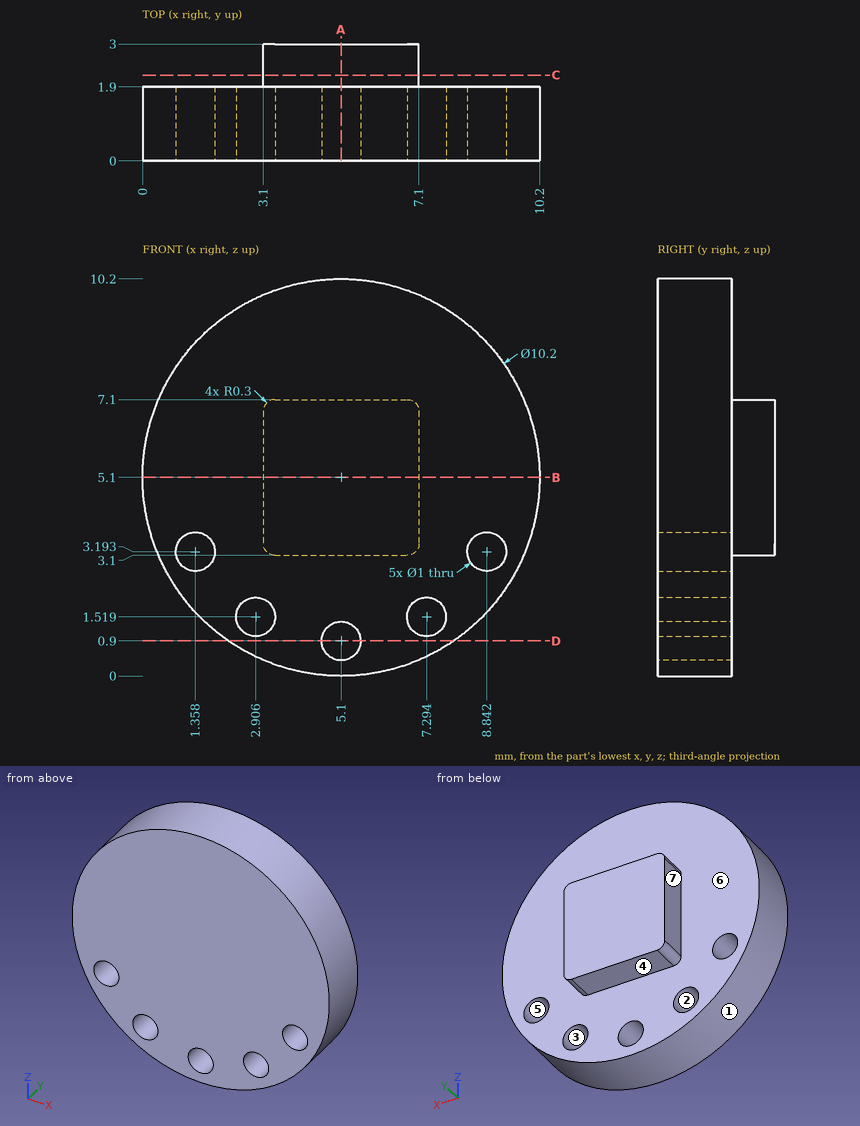
The figure shows three views and two pictorial views of one solid part (mm, origin at its lowest corner). Answer the questions. A direction names the side the tool comes from. Round coordinates to 2 decimals unless told otherwise and drop trailing zeros. Write each loop counter-clockwise with the first axis right and the second up, starting at its lowest first coordinate (ties: lowest second). Pieces come first, ordered by that corner, then holes. Notation, with made-up numbers: M 87,-2 L 136,-2 A13 cw 136,19 Z; hole C 83.25,8.25 d1. An arc over 180 degrees is marked long. Use a Markdown table: item, result.
1) A flat-ended cylindrical pin translates along its axis: pin 1 (1.5 mm diameter, centred on x = 4, y = 2.5, fed in from +Z). Find the tip coordinate at first contact, or state that the pin passes through.
Taken from the geometry:
| item | result |
|---|---|
| pin 1 | stops at z = 10.16 |
2) Consider line 1 (X direction, y = 0.7, z = 3) (1 decimal); line 2 (X direction, y = 2.2, z = 5.75); line 3 (Y direction, x = 7.75, z = 8.5). Determine where each line is inside the solid, lowest interval first. Write a range as [from, to].
Taken from the geometry:
| item | result |
|---|---|
| line 1 | x = [0.5, 0.9], [1.8, 8.4], [9.3, 9.7] |
| line 2 | x = [3.1, 7.1] |
| line 3 | y = [0, 1.9] |
3) Determine the mould class of the marked faces 1, 2, 3 and 4 for opening direction Z: pulls with the +Z half, pulls with the -Z half, needs draft (parallel to the pull), parting line crosses it, or undercut.
Taken from the geometry:
| item | result |
|---|---|
| face 1 | parting line crosses it |
| face 2 | undercut |
| face 3 | undercut |
| face 4 | pulls with the -Z half |
4) The part is cut by section C-C on y = 2.2. Give the vertices of the cut face in (x, z), plus the area to 3 significant figures.
Taken from the geometry:
| item | result |
|---|---|
| outline | M 3.1,3.4 A0.3 ccw 3.4,3.1 L 6.8,3.1 A0.3 ccw 7.1,3.4 L 7.1,6.8 A0.3 ccw 6.8,7.1 L 3.4,7.1 A0.3 ccw 3.1,6.8 Z |
| area | 15.9 mm2 |
5) Which of the six approach directions +Z, -Z, +X, -X, +Y, -Y give full straight-line access (tool end or side, diameter ignored) to the marked faces 5, 6 and 7?
Taken from the geometry:
| item | result |
|---|---|
| face 5 | +Y, -Y |
| face 6 | +Y |
| face 7 | +Z, -Z, -X, +Y |
6) The part is cut by section B-B on z = 5.1. Give the vertices of the cut face in (x, y).
Taken from the geometry:
| item | result |
|---|---|
| outline | M 0,0 L 10.2,0 L 10.2,1.9 L 7.1,1.9 L 7.1,3 L 3.1,3 L 3.1,1.9 L 0,1.9 Z |
7) The part is cut by section A-A on x = 5.1. Give the vertices of the cut face in (y, z), plus the area to 3 significant figures.
Taken from the geometry:
| item | result |
|---|---|
| outline | M 0,0 L 1.9,0 L 1.9,0.4 L 0,0.4 Z; M 0,1.4 L 1.9,1.4 L 1.9,3.1 L 3,3.1 L 3,7.1 L 1.9,7.1 L 1.9,10.2 L 0,10.2 Z |
| area | 21.9 mm2 |
8) The part is cut by section D-D on z = 0.9. Give the vertices of the cut face in (x, y).
Taken from the geometry:
| item | result |
|---|---|
| outline | M 2.21,0 L 4.6,0 L 4.6,1.9 L 2.21,1.9 Z; M 5.6,0 L 7.99,0 L 7.99,1.9 L 5.6,1.9 Z |
